from build123d import *

# Parameters (mm, degrees)
F1_DEPTH = 1100


with BuildPart() as f1:
    # F0 (on Front) → F1 (new body)
    with BuildSketch(Plane.XZ):
        Polygon((5, -20), (20, -20), (20, -5), (15, -5), (15, -10), (10, -5), (10, 5), (15, 10), (15, 5), (20, 5), (20, 20), (20, 35), (15, 35), (15, 30), (10, 35), (10, 45), (15, 50), (15, 45), (20, 45), (20, 60), (5, 60), (5, 55), (10, 55), (5, 50), (-5, 50), (-10, 55), (-5, 55), (-5, 60), (-20, 60), (-20, 45), (-15, 45), (-15, 50), (-10, 45), (-10, 35), (-15, 30), (-15, 35), (-20, 35), (-20, 20), (-20, 5), (-15, 5), (-15, 10), (-10, 5), (-10, -5), (-15, -10), (-15, -5), (-20, -5), (-20, -20), (-5, -20), (-5, -15), (-10, -15), (-5, -10), (5, -10), (10, -15), (5, -15), align=None)
        Polygon((-5, 0), (-5, 5), (0, 5), (5, 5), (5, 0), (5, -5), (0, -5), (-5, -5), align=None, mode=Mode.SUBTRACT)
        Polygon((-5, 15), (-5, 20), (-5, 25), (-10, 25), (-5, 30), (5, 30), (10, 25), (5, 25), (5, 20), (5, 15), (10, 15), (5, 10), (-5, 10), (-10, 15), align=None, mode=Mode.SUBTRACT)
        Polygon((-5, 40), (-5, 45), (0, 45), (5, 45), (5, 40), (5, 35), (0, 35), (-5, 35), align=None, mode=Mode.SUBTRACT)
    extrude(amount=F1_DEPTH)


solid = f1.part
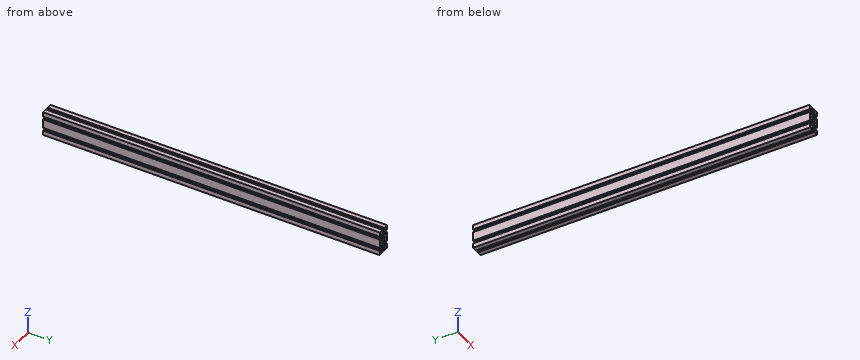
Source: CAD feature listing. Evaluate the final solid. Frame: model axes, mm. Round coordinates to 2 decimals unless told otherwise and drop trailing zeros. Write item = value, one per line. Start each with the question number.
Item 1: First-contact query: pin 1 Ø5 at (x, y) = (2, -738) entering from +Z; pin 2 Ø5 at (y, z) = (-694.5, 40) entering from -X. Flat tips, straight axial feed; report the tip coordinate or a pass-through.
Item 2: Material intervals for line 1 (Z direction, x = 3, y = -1005); line 2 (X direction, y = -494, z = 39); line 3 (Z direction, x = -9, y = -177), sorted ascending.
Item 3: Section query A-A on y = -524.5. Count the separate pieces of the cut face and the enclosed holes in it, plus the area to 3 significant figures.
Results list:
q1.pin_1 = 50
q1.pin_2 = -10
q2.line_1 = -10 to -5, 5 to 10, 30 to 35, 45 to 50
q2.line_2 = -10 to -5, 5 to 10
q2.line_3 = -20 to -15, -14 to 14, 15 to 25, 26 to 54, 55 to 60
q3.separate_pieces = 1
q3.enclosed_holes = 3
q3.area = 2,000 mm²
